Part model, mm, in its own coordinate system. A direction names the side the tool comes from. Give positions to 0.01 mm unless a question says otherwise; leave off trailing zeros. Write each loop counter-clockwise with the first axis right and the second up, starting at its lowest first coordinate (ties: lowest second). Pieces come first, ordered by that corner, then holes. Notation, with made-up numbers: M -2,-5.5 L 26,-5.5 A33 ccw 26,23.5 Z; hole C -13.75,64.5 d2. An arc over 180 degrees is marked long. Answer as CSV lines item,"result". Start each with the question number.
Item 1: Band-saw the part on D-D, the plane z = -8. List the corners of the cut face in (x, y), then the cut area to 3 significant figures.
Item 2: Pin check, flat tips, straight feed: pin 1 (1.5 mm diameter, centred on y = 9.5, z = 11, fed in from +X); pin 2 (6.5 mm diameter, centred on x = 1, y = 9.5, fed in from +Z); pin 3 (5 mm diameter, centred on x = 3.5, y = 10, fed in from -Z); pin 4 (2 mm diameter, centred on x = 0, y = 8, fed in from +Z). Stop position of each tip, or through.
Item 3: Band-saw the part on B-B, the plane y = 19.75. List the corners of the cut face in (x, z).
Item 4: Wall check: L1, parallel to X at y = 9.75, z = -20; L2, parallel to Z at x = 5.5, y = 13; L3, parallel to Z at x = -5, y = 19.75. Give the ranges that are in metal, low to high. Write a range as from..to.
Item 5: 3-axis set-ups, long thin cutter, end or side, ignore diameter. For faces 4 (the flat face through (8.2, 8.9, -27.4)), 5 (the flat face through (0, 19, 0)), 6 (the flat face through (6.2, 14, -8)), 7 (the cylindrical face through (-0.54, 5.56, 7.15)): which of +Z, -Z, +X, -X, +Y, -Y reach the whole face in a straight line?
Item 6: Two-plate mould, pull along X, no slides. Class faces 1 (the flat face through (0, 14, -1.8)), 2 (the flat face through (-8, 19, -8)), 3 (the flat face through (0, 0, -8)): +X half, -X half, draft (parallel to the pull), parting line (faces both ways), or undercut.
Item 7: Band-saw the part on A-A, the plane y = 8. List the corners of the cut face in (x, z).
Item 8: Band-saw the part on C-C, the plane x = 0. Count the separate pieces of the cut face and the enclosed holes in it, then the cut area to 3 significant figures.
from build123d import *

# Parameters (mm, degrees)
SKETCH1_W           = 16
SKETCH1_H           = 16
BOSS_EXTRUDE1_DEPTH = 24
SKETCH12_W          = 12.4
SKETCH12_H          = 12.4
CUT_EXTRUDE6_DEPTH  = 22
SKETCH13_R          = 25
BOSS_EXTRUDE2_DEPTH = 3
CHAMFER1_SIZE       = 2.5
SKETCH14_W          = 18
SKETCH14_H          = 40.4
SKETCH14_W_2        = 16
SKETCH14_H_2        = 16
BOSS_EXTRUDE3_DEPTH = 12
CHAMFER2_SIZE       = 1.6
CHAMFER5_SIZE       = 1
SKETCH16_W          = 12
SKETCH16_H          = 8
CUT_EXTRUDE8_DEPTH  = 14
SKETCH15_R          = 1.3
CUT_EXTRUDE7_DEPTH  = 19.8
SKETCH17_R          = 2.5
CUT_EXTRUDE9_DEPTH  = 9
SKETCH19_R          = 3
CUT_EXTRUDE10_DEPTH = 1.2


with BuildPart() as part:
    # Sketch1 → Boss-Extrude1 (new body)
    with BuildSketch(Plane(origin=(0, 0, 0), x_dir=(1, 0, 0), z_dir=(0, 1, 0))):
        with Locations((0, 8)):
            Rectangle(SKETCH1_W, SKETCH1_H)
    extrude(amount=BOSS_EXTRUDE1_DEPTH)

    # Sketch12 → Cut-Extrude6 (cut)
    with BuildSketch(Plane(origin=(0, 24, 0), x_dir=(1, 0, 0), z_dir=(0, 1, 0))):
        with Locations((0, 8)):
            Rectangle(SKETCH12_W, SKETCH12_H)
    extrude(amount=-CUT_EXTRUDE6_DEPTH, mode=Mode.SUBTRACT)

    # Sketch13 → Boss-Extrude2 (add)
    with BuildSketch(Plane(origin=(0, 0, 0), x_dir=(1, 0, 0), z_dir=(0, 1, 0))):
        with Locations((0, 8)):
            Circle(SKETCH13_R)
    extrude(amount=BOSS_EXTRUDE2_DEPTH)

    # Chamfer1
    chamfer1_edges = [part.edges().sort_by_distance(p)[0] for p in [
        (-25, 3, -8),
    ]]
    chamfer(chamfer1_edges, length=CHAMFER1_SIZE)

    # Sketch14 → Boss-Extrude3 (add)
    with BuildSketch(Plane(origin=(0, 3, 0), x_dir=(1, 0, 0), z_dir=(0, 1, 0))):
        with Locations((0, 8)):
            Rectangle(SKETCH14_W, SKETCH14_H)
        with Locations((0, 8)):
            Rectangle(SKETCH14_W_2, SKETCH14_H_2, mode=Mode.SUBTRACT)
    extrude(amount=BOSS_EXTRUDE3_DEPTH)

    # Chamfer2
    chamfer2_edges = [part.edges().sort_by_distance(p)[0] for p in [
        (0, 15, 12.2),
        (0, 15, -28.2),
        (-9, 9, 12.2),
        (9, 9, 12.2),
        (9, 9, -28.2),
        (-9, 9, -28.2),
    ]]
    chamfer(chamfer2_edges, length=CHAMFER2_SIZE)

    # Chamfer5
    chamfer5_edges = [part.edges().sort_by_distance(p)[0] for p in [
        (0, 24, -16),
        (-8, 24, -8),
        (0, 24, 0),
        (8, 24, -8),
    ]]
    chamfer(chamfer5_edges, length=CHAMFER5_SIZE)

    # Sketch16 → Cut-Extrude8 (cut)
    with BuildSketch(Plane(origin=(0, 0, -28.2), x_dir=(-1, 0, 0), z_dir=(0, 0, -1))):
        with Locations((0, 8)):
            Rectangle(SKETCH16_W, SKETCH16_H)
    extrude(amount=-CUT_EXTRUDE8_DEPTH, mode=Mode.SUBTRACT)

    # Sketch15 → Cut-Extrude7 (cut, through all)
    with BuildSketch(Plane(origin=(0, 0, -1.8), x_dir=(-1, 0, 0), z_dir=(0, 0, -1))):
        with Locations((0, 8)):
            Circle(SKETCH15_R)
    extrude(amount=-CUT_EXTRUDE7_DEPTH, mode=Mode.SUBTRACT)

    # Sketch17 → Cut-Extrude9 (cut)
    with BuildSketch(Plane.XY.offset(12.2)):
        with Locations((0, 8)):
            Circle(SKETCH17_R)
    extrude(amount=-CUT_EXTRUDE9_DEPTH, mode=Mode.SUBTRACT)

    # Sketch19 → Cut-Extrude10 (cut)
    with BuildSketch(Plane.XY.offset(12.2)):
        with Locations((0, 8)):
            Circle(SKETCH19_R)
    extrude(amount=-CUT_EXTRUDE10_DEPTH, mode=Mode.SUBTRACT)


solid = part.part
Output:
1,outline,"M -25,0 L 25,0 L 25,0.5 L 22.5,3 L 9,3 L 9,15 L 8,15 L 8,23 L 7,24 L 6.2,24 L 6.2,3 L -6.2,3 L -6.2,24 L -7,24 L -8,23 L -8,15 L -9,15 L -9,3 L -22.5,3 L -25,0.5 Z"
1,area,"242 mm²"
2,pin 1,"x = 9"
2,pin 2,"z = 12.2"
2,pin 3,"z = -28.2"
2,pin 4,"through"
3,outline,"M -8,-16 L 8,-16 L 8,0 L -8,0 Z; hole M -6.2,-14.2 L 6.2,-14.2 L 6.2,-1.8 L -6.2,-1.8 Z"
4,L1,"-9..-6, 6..9"
4,L2,"-28.2..-14.2, -1.8..12.2"
4,L3,"-16..-14.2, -1.8..0"
5,face 4,"-Z, +X, +Y"
5,face 5,"+Z, +X, -X, +Y"
5,face 6,"+Y"
5,face 7,"+Z"
6,face 1,"undercut"
6,face 2,"-X half"
6,face 3,"draft"
7,outline,"M -9,-26.6 L -7.4,-28.2 L -6,-28.2 L -6,-14.2 L -6.2,-14.2 L -6.2,-1.8 L -1.3,-1.8 L -1.3,3.2 L -2.5,3.2 L -2.5,11 L -3,11 L -3,12.2 L -7.4,12.2 L -9,10.6 Z; M 1.3,-1.8 L 6.2,-1.8 L 6.2,-14.2 L 6,-14.2 L 6,-28.2 L 7.4,-28.2 L 9,-26.6 L 9,10.6 L 7.4,12.2 L 3,12.2 L 3,11 L 2.5,11 L 2.5,3.2 L 1.3,3.2 Z"
8,separate pieces,"3"
8,enclosed holes,"0"
8,area,"337 mm²"
